Verification items for the finished model (mm, model axes). Face numbers are marked on the shaded views. A direction names the side the tool comes from. Give positions to 0.01 mm unless a question says otherwise; leave off trailing zeros. Write each loop counter-clockwise with the first axis right and the second up, starting at its lowest first coordinate (ties: lowest second). Pieces come first, ordered by that corner, then holes. Notation, with made-up numbers: (35.5, -9.75) -> (57.5, -9.75) arc R22 cw to (57.5, 3.25) -> close; hole circle Ø3 at (-4.75, 30.5). An arc over 180 degrees is marked (long way). Write item = value, one per line.
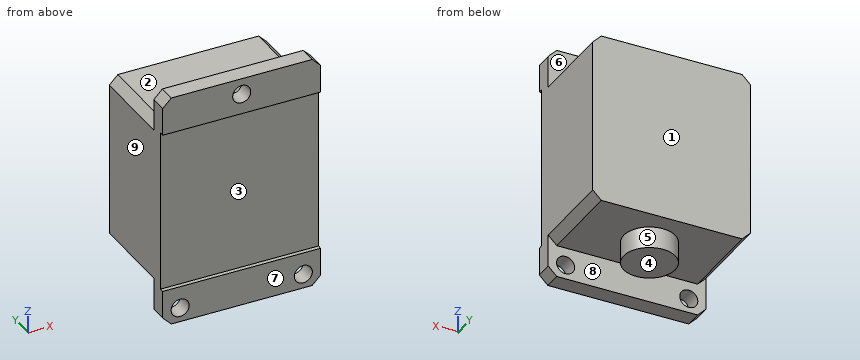
from build123d import *

# Parameters (mm, degrees)
SKETCH3_W           = 36.8
SKETCH3_H           = 55
BOSS_EXTRUDE2_DEPTH = 24
SKETCH4_W           = 38
SKETCH4_H           = 1
SKETCH4_W_2         = 7.5
SKETCH4_H_2         = 20
CUT_EXTRUDE1_DEPTH  = 37.8
SKETCH5_R           = 2.1
CUT_EXTRUDE2_DEPTH  = 5
CHAMFER1_SIZE       = 2
SKETCH6_R           = 6
BOSS_EXTRUDE3_DEPTH = 5


with BuildPart() as part:
    # Sketch3 → Boss-Extrude2 (new body)
    with BuildSketch(Plane(origin=(0, 0, 0), x_dir=(1, 0, 0), z_dir=(0, 1, 0))):
        with Locations((18.4, 27.5)):
            Rectangle(SKETCH3_W, SKETCH3_H)
    extrude(amount=BOSS_EXTRUDE2_DEPTH)

    # Sketch4 → Cut-Extrude1 (cut, through all)
    with BuildSketch(Plane(origin=(36.8, 0, 0), x_dir=(0, 0, -1), z_dir=(1, 0, 0))):
        with Locations((27.5, 0.5)):
            Rectangle(SKETCH4_W, SKETCH4_H)
        with Locations((51.25, 14)):
            Rectangle(SKETCH4_W_2, SKETCH4_H_2)
        with Locations((3.75, 14)):
            Rectangle(SKETCH4_W_2, SKETCH4_H_2)
    extrude(amount=-CUT_EXTRUDE1_DEPTH, mode=Mode.SUBTRACT)

    # Sketch5 → Cut-Extrude2 (cut, through all)
    with BuildSketch(Plane(origin=(0, 4, 0), x_dir=(1, 0, 0), z_dir=(0, 1, 0))):
        with Locations((18.4, 3.75)):
            Circle(SKETCH5_R)
        with Locations((32.75, 51.65)):
            Circle(SKETCH5_R)
        with Locations((4.05, 51.65)):
            Circle(SKETCH5_R)
    extrude(amount=-CUT_EXTRUDE2_DEPTH, mode=Mode.SUBTRACT)

    # Chamfer1
    chamfer1_edges = [part.edges().sort_by_distance(p)[0] for p in [
        (0, 2, -55),
        (36.8, 2, -55),
        (36.8, 2, 0),
        (0, 2, 0),
        (0, 14, -47.5),
        (36.8, 14, -47.5),
        (0, 14, -7.5),
        (36.8, 14, -7.5),
    ]]
    chamfer(chamfer1_edges, length=CHAMFER1_SIZE)

    # Sketch6 → Boss-Extrude3 (add)
    with BuildSketch(Plane(origin=(0, 0, -47.5), x_dir=(-1, 0, 0), z_dir=(0, 0, -1))):
        with Locations((-18.4, 14)):
            Circle(SKETCH6_R)
    extrude(amount=BOSS_EXTRUDE3_DEPTH)


solid = part.part
Item 1: Material ranges on line 1 (X direction, y = 0.8, z = -51.65); line 2 (Z direction, x = 32.75, y = 2.2); line 3 (Z direction, x = 18.4, y = 2.7), recorded low to high.
Response values:
line_1 = 0 to 1.95, 6.15 to 30.65, 34.85 to 36.8
line_2 = -55 to -53.75, -49.55 to 0
line_3 = -55 to -5.85, -1.65 to 0
Item 2: Sectioned sample at B-B on z = -51.65. Record the cut outline in (x, y).
Response values:
outline = (0, 0) -> (1.95, 0) -> (1.95, 4) -> (0, 4) -> close; (6.15, 0) -> (30.65, 0) -> (30.65, 4) -> (6.15, 4) -> close; circle Ø12 at (18.4, 14); (34.85, 0) -> (36.8, 0) -> (36.8, 4) -> (34.85, 4) -> close
Item 3: Sectioned sample at C-C on x = 18.4. Record the cut outline in (y, z).
Response values:
outline = (0, -55) -> (4, -55) -> (4, -47.5) -> (8, -47.5) -> (8, -52.5) -> (20, -52.5) -> (20, -47.5) -> (24, -47.5) -> (24, -7.5) -> (4, -7.5) -> (4, -5.85) -> (0, -5.85) -> (0, -8.5) -> (1, -8.5) -> (1, -46.5) -> (0, -46.5) -> close; (0, -1.65) -> (4, -1.65) -> (4, 0) -> (0, 0) -> close
Item 4: Sectioned sample at A-A on y = 2.5. Record the cut outline in (x, z), then the cut area to 3 significant figures.
Response values:
outline = (0, -53) -> (2, -55) -> (34.8, -55) -> (36.8, -53) -> (36.8, -2) -> (34.8, 0) -> (2, 0) -> (0, -2) -> close; hole circle Ø4.2 at (4.05, -51.65); hole circle Ø4.2 at (18.4, -3.75); hole circle Ø4.2 at (32.75, -51.65)
area = 1,970 mm^2
Item 5: Set-up check for the marked faces 1, 2, 3, 4 and 5: record each of +Z, -Z, +X, -X, +Y, -Y from which the full face is reachable in a straight line by a thin tool's end or side.
Response values:
face_1 = +Z, -Z, +X, -X, +Y
face_2 = +Z, +X, -X, +Y
face_3 = +X, -X, -Y
face_4 = -Z, +X, -X, +Y
face_5 = -Z
Item 6: Go/stop test with flat-tipped pins: P1, Ø3.5, axis at x = 19, y = 12, coming from the -Z side; P2, Ø10, axis at x = 18.5, y = 11.5, coming from the +Z side; P3, Ø5, axis at x = 15, z = -51.5, coming from the +Y side. Record where each tip stops, or that it passes through.
Response values:
P1 = -52.5
P2 = -7.5
P3 = 19.93
Item 7: Sectioned sample at D-D on y = 14. Record the cut outline in (x, z).
Response values:
outline = (0, -45.5) -> (2, -47.5) -> (12.4, -47.5) -> (12.4, -52.5) -> (24.4, -52.5) -> (24.4, -47.5) -> (34.8, -47.5) -> (36.8, -45.5) -> (36.8, -9.5) -> (34.8, -7.5) -> (2, -7.5) -> (0, -9.5) -> close
Item 8: Mould release check, pull along Y, two halves, no side actions. Record for the marked faces 6, 7, 8 and 9: +Y half, -Y half, draft (parallel to the pull), parting line (faces both ways), or undercut.
Response values:
face_6 = +Y half
face_7 = -Y half
face_8 = undercut
face_9 = draft
